Work out the finished part from the listing and answer in its coordinate system (mm). A direction names the side the tool comes from. Coordinates: 2 decimals unless noted, no trailing zeros. Order: outer loops, then holes, each group sorted by start corner. A loop starts at its lowest first (then second) coordinate and runs counter-clockwise, first axis right, second up. Notation, with made-up numbers: M 5,49 L 38,49 A36 cw 38,84 Z; hole C 10.5,24.5 d11. An arc over 180 degrees is marked long. Write item = value, one per line. Start each with the question number.
Q1. A tool of negligible diameter and unlimited length cuts with its end or side. For faces 4 (the flat face through (56, -76, -19)), 5 (the flat face through (-1, -37, -25)), 6 (the flat face through (30, 0, -19)), 7 (the flat face through (55, -77, -19)), from which of +Z, -Z, +X, -X, +Y, -Y can it reach the whole face along a straight path? Write none if from no direction.
Q2. Find section C-C on x = 24. Give the vertices of the cut face in (y, z).
Q3. Determine the mould class of faces 1 (the flat face through (-8, -76, -19)), 2 (the cylindrical face through (17.506, 0.507, -25.286)), 3 (the cylindrical face through (60.491, -76.493, -32.684)) for opening direction Z: released by +Z, released by -Z, zero draft, split by the parting line, or undercut.
Q4. Find section A-A on z = -25. Give the vertices of the cut face in (x, y).
Q5. Find section D-D on z = -8.5. Give the vertices of the cut face in (x, y), and give its area (3 significant figures).
Q6. Each of these flat-tipped pins is pushed along its axis until it touches: P1, Ø3, axis at y = -14.5, z = -29, coming from the +X side; P2, Ø4, axis at y = -11.5, z = -24.5, coming from the -X side; P3, Ø5, axis at x = 17, z = -40.5, coming from the -Y side; P4, Ø9.5, axis at x = 61.5, z = -25, coming from the +Y side. Where does it stop, or does it pass through?
Q7. Find section B-B on y = -39. Give the vertices of the cut face in (x, z).
Q8. Straight lines are drawn through the part: line 1 along X through (y, z) = (-76.7, -25); line 2 along Z through (x, y) = (-13.5, -76.8); line 3 along X through (y, z) = (-24, -45.5). For each, find the intervals that lie inside material, in ascending order.
Autodesk Inventor part; units mm, degrees
ref_plane "YZ Plane" through (0, 0, 0) normal (1, 0, 0) x (0, 1, 0)
ref_plane "XZ Plane" through (0, 0, 0) normal (0, 1, 0) x (-1, 0, 0)
ref_plane "XY Plane" through (0, 0, 0) normal (0, 0, 1) x (1, 0, 0)
sketch "Sketch1" plane through (0, 0, 0) normal (0, 1, 0) x (-1, 0, 0)
  line L0 (0, 0) -> (-48, 0)
  line L1 (-48, 0) -> (-48, -50)
  line L2 (-48, -50) -> (0, -50)
  line L3 (0, -50) -> (0, 0)
  dimension "d0" = 48
  dimension "d1" = 50
extrude "Extrusion1" add sketch "Sketch1" along normal blind 1
sketch "Sketch2" plane through (48, 0, 0) normal (1, 0, 0) x (0, 0, -1)
  line L0 (0, 1) -> (50, 1)
  line L1 (0, 1) -> (50, 1)
  line L2 (50, 1) -> (50, -76)
  line L3 (50, -76) -> (0, -76)
  line L4 (0, -76) -> (0, 1)
  point P0 (0, 0)
  dimension "d4" = 50
  dimension "d5" = 77
extrude "Extrusion2" add sketch "Sketch2" along normal blind 1
sketch "Sketch3" plane through (0, 0, -50) normal (-1, 0, 0) x (0, 0, 1)
  line L0 (0, 0) -> (0, 1)
  line L1 (50, 0) -> (50, -76)
  line L2 (0, 1) -> (50, 1)
  line L3 (50, 1) -> (50, -76)
  line L4 (50, -76) -> (0, -76)
  line L5 (0, -76) -> (0, 1)
extrude "Extrusion3" add sketch "Sketch3" along normal blind 1
sketch "Sketch4" plane through (0, 1, 0) normal (0, 1, 0) x (1, 0, 0)
  point P0 (0, 0)
sketch "Sketch5" plane through (0, -76, -50) normal (0, -1, 0) x (1, 0, 0)
  line L0 (0, 50) -> (-26, 50)
  line L1 (-26, 50) -> (-26, 0)
  line L2 (-26, 0) -> (0, 0)
  line L3 (0, 0) -> (0, 50)
  line L4 (48, 50) -> (48, 0)
  line L5 (48, 50) -> (74, 50)
  line L6 (74, 50) -> (74, 0)
  line L7 (74, 0) -> (48, 0)
  line L8 (48, 0) -> (48, 50)
  dimension "d10" = 26
  dimension "d11" = 26
extrude "Extrusion4" add sketch "Sketch5" along normal blind 1
sketch "Sketch6" plane through (0, 1, 0) normal (0, 1, 0) x (1, 0, 0)
  circle A0 centre (24, 25) radius 6.5
  line L0 (-1, 50) -> (49, 50)
  line L1 (49, 50) -> (49, 0)
  line L2 (49, 50) -> (74, 50)
  line L3 (74, 50) -> (74, 0)
  line L4 (-26, 50) -> (-1, 50)
  line L5 (-26, 0) -> (-26, 50)
  point P0 (0, 0)
  dimension "d14" = 13
  dimension "d17" = 25
  dimension "d18" = 25
extrude "Extrusion5" cut sketch "Sketch6" against normal blind 1
sketch "Sketch7" plane through (0, -76, -50) normal (0, 1, 0) x (1, 0, 0)
  circle A0 centre (61.5, -25) radius 7.75
  circle A1 centre (-13.5, -25) radius 7.75
  line L0 (-26, 0) -> (-1, 0)
  line L1 (-26, -50) -> (-26, 0)
  line L2 (74, 0) -> (74, -50)
  line L3 (49, 0) -> (74, 0)
  point P0 (0, -50)
  dimension "d25" = 15.5
  dimension "d26" = 15.5
  dimension "d27" = 25
  dimension "d28" = 12.5
  dimension "d29" = 12.5
  dimension "d30" = 25
extrude "Extrusion6" cut sketch "Sketch7" against normal blind 15.5
equation "\"d31\" = d25"
properties part number "cla3" material "Iron, Cast"
Findings below:
q1.face_4 = +Z, -Z, +X, +Y
q1.face_5 = +Z, -Z, -X, +Y
q1.face_6 = +Z, -Z, -Y
q1.face_7 = +Z, -Z, +X, -X, -Y
q2.outline = M 0,-50 L 1,-50 L 1,-31.5 L 0,-31.5 Z; M 0,-18.5 L 1,-18.5 L 1,0 L 0,0 Z
q3.face_1 = zero draft
q3.face_2 = undercut
q3.face_3 = undercut
q4.outline = M -26,-77 L -21.25,-77 L -21.25,-76 L -26,-76 Z; M -5.75,-77 L 0,-77 L 0,0 L 17.5,0 L 17.5,1 L -1,1 L -1,-76 L -5.75,-76 Z; M 30.5,0 L 48,0 L 48,-77 L 53.75,-77 L 53.75,-76 L 49,-76 L 49,1 L 30.5,1 Z; M 69.25,-77 L 74,-77 L 74,-76 L 69.25,-76 Z
q5.outline = M -26,-77 L 0,-77 L 0,0 L 48,0 L 48,-77 L 74,-77 L 74,-76 L 49,-76 L 49,1 L -1,1 L -1,-76 L -26,-76 Z
q5.area = 254 mm^2
q6.P1 = 49
q6.P2 = -1
q6.P3 = 0
q6.P4 = through
q7.outline = M -1,-50 L 0,-50 L 0,0 L -1,0 Z; M 48,-50 L 49,-50 L 49,0 L 48,0 Z
q8.line_1 = -26 to -21.25, -5.75 to 0, 48 to 53.75, 69.25 to 74
q8.line_2 = -50 to -32.75, -17.25 to 0
q8.line_3 = -1 to 0, 48 to 49
